Geometry check sheet. Reference: drawing and pictorial views, mm from the part's lowest x, y, z. Coordinates: 2 decimals unless noted, no trailing zeros. Write each loop counter-clockwise with the first axis right and the second up, starting at its lowest first coordinate (ties: lowest second). Pieces come first, ordered by that corner, then holes. Notation, with made-up numbers: (32.25, 80.25) - (58.25, 80.25) arc R34 ccw to (58.25, 112.25) - close; hole circle Ø6 at (-35.75, 86). An arc over 180 degrees is marked (long way). Use one line per item in the form item = value. Start each with the question number.
(1) Material ranges on line 1 (Y direction, x = 602, z = 1492); line 2 (X direction, y = 393, z = 183.5); line 3 (Z direction, x = 37.5, y = 576), recorded low to high. Write a range as [from, to].
(2) Gauge pin test, flat end, axial feed: pin 1 Ø2 at (x, y) = (459.5, 411.5) entering from -Z. Record the tip position at first contact, or that the pin passes through.
(3) Sectioned sample at C-C (y = 420). Record the cut outline in (x, z), and give its area (3 significant figures).
(4) Sectioned sample at A-A (z = 1451.5). Record the cut outline in (x, y), and give its area (3 significant figures).
(5) Sectioned sample at B-B (y = 261.5). Record the cut outline in (x, z).
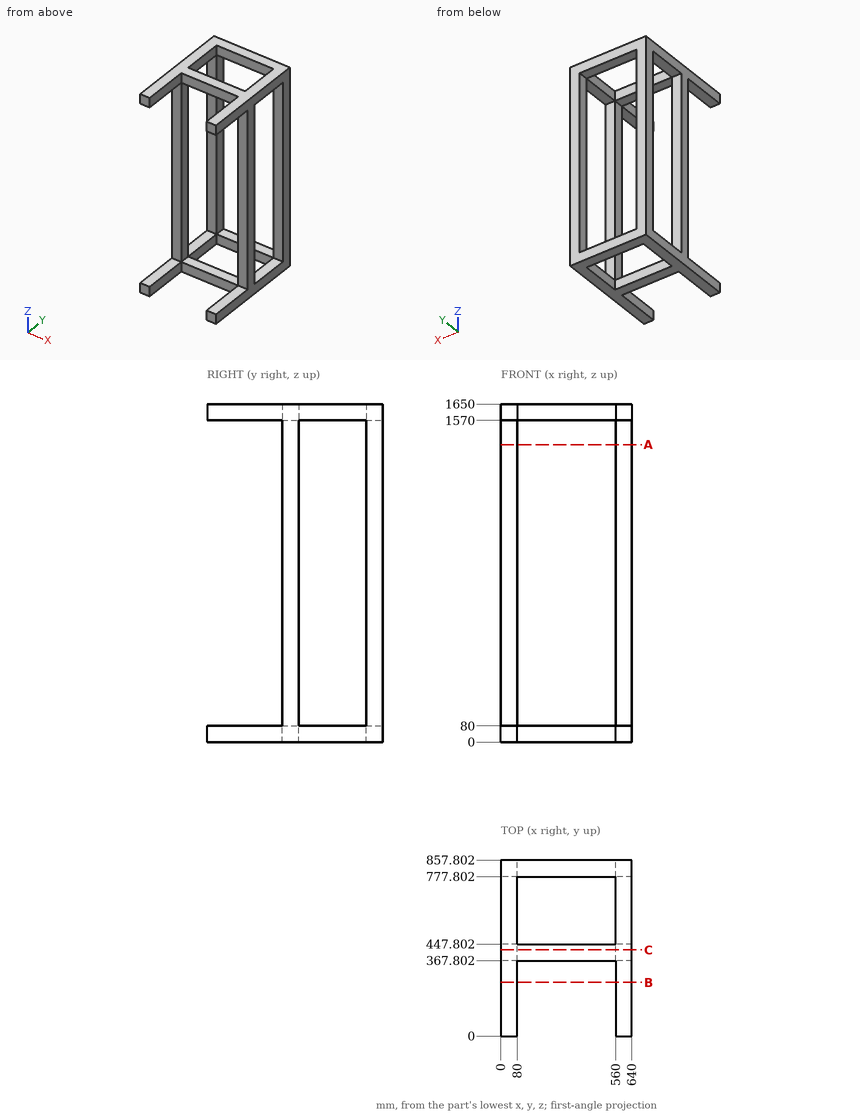
Answers below:
q1.line_1 = [367.8, 447.8], [777.8, 857.8]
q1.line_2 = [0, 80], [560, 640]
q1.line_3 = [0, 80], [1570, 1650]
q2.pin_1 = 0
q3.outline = (0, 0) - (640, 0) - (640, 1650) - (0, 1650) - close; hole (80, 80) - (560, 80) - (560, 1570) - (80, 1570) - close
q3.area = 341,000 mm2
q4.outline = (0, 367.8) - (80, 367.8) - (80, 447.8) - (0, 447.8) - close; (0, 777.8) - (80, 777.8) - (80, 857.8) - (0, 857.8) - close; (560, 367.8) - (640, 367.8) - (640, 447.8) - (560, 447.8) - close; (560, 777.8) - (640, 777.8) - (640, 857.8) - (560, 857.8) - close
q4.area = 25,600 mm2
q5.outline = (0, 0) - (80, 0) - (80, 80) - (0, 80) - close; (0, 1570) - (80, 1570) - (80, 1650) - (0, 1650) - close; (560, 0) - (640, 0) - (640, 80) - (560, 80) - close; (560, 1570) - (640, 1570) - (640, 1650) - (560, 1650) - close
